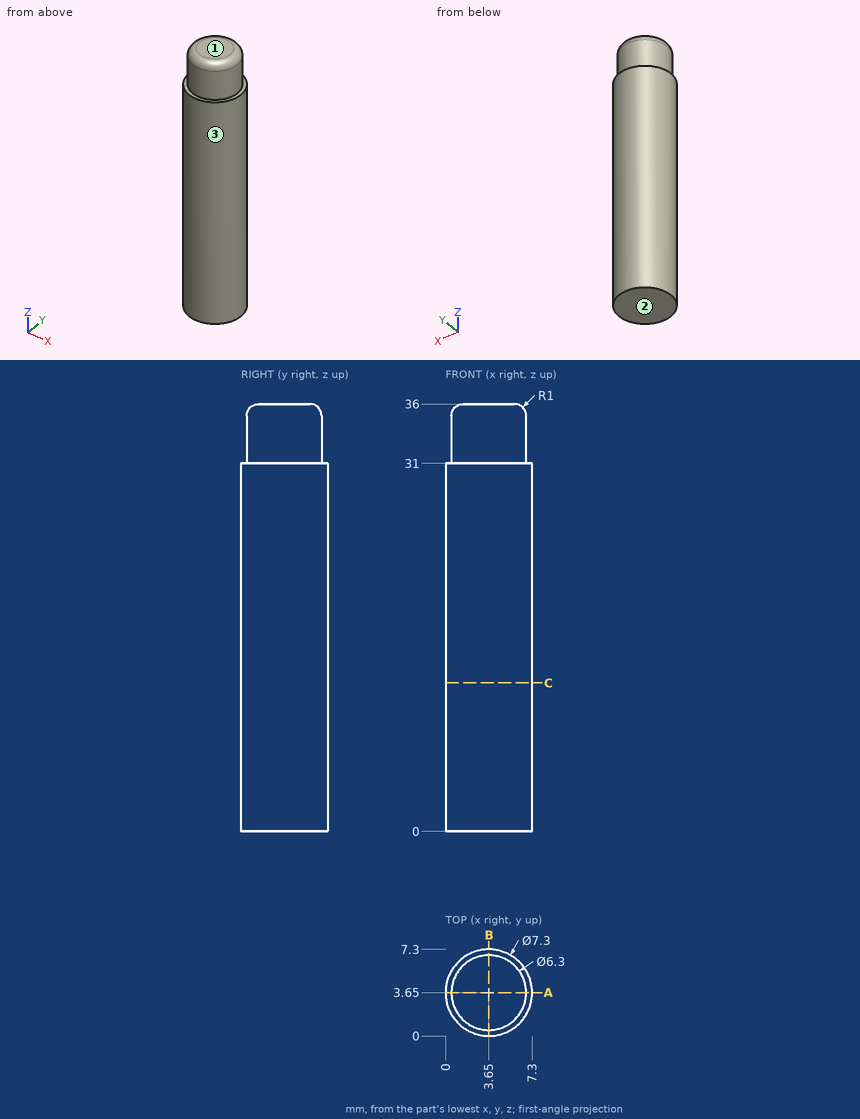
Print and shaded views of the part. All mm, measured from the part's lowest x, y and z. Give positions to 0.01 mm unless a question says otherwise; leave off trailing zeros. Loops run counter-clockwise (first coordinate to the right, second up) from the corner with the lowest first, then second, coordinate; pieces in that order, holes last. Notation, with made-up numbers: (3.25, 14) -> (10.25, 14) arc R6 ccw to (10.25, 20) -> close; hole circle Ø5 at (-30.75, 4.5). An arc over 180 degrees is marked (long way). One line per question, with ' | ' between items. Start each with the question number.
1) Two-plate mould, pull along Z, no slides. Class the marked faces 1, 2 and 3: released by +Z, released by -Z, zero draft, split by the parting line, or undercut.
2) Probe L1, parallel to Y at x = 3.75, z = 27; L2, parallel to Z at x = 1.25, y = 6; L3, parallel to Y at x = 1.5, z = 3. List the from-to ranges inside material, lowest first.
3) Cut at C-C (z = 12.5). Give the cut face in (x, y), plus the area to 3 significant figures.
4) Cut at A-A (y = 3.65). Give the cut face in (x, z), plus the area to 3 significant figures.
Return value:
1) face 1: released by +Z | face 2: released by -Z | face 3: zero draft
2) L1: 0 to 7.3 | L2: 0 to 31 | L3: 0.7 to 6.6
3) outline: circle Ø7.3 at (3.65, 3.65) | area: 41.9 mm^2
4) outline: (0, 0) -> (7.3, 0) -> (7.3, 31) -> (6.8, 31) -> (6.8, 35) arc R1 ccw to (5.8, 36) -> (1.5, 36) arc R1 ccw to (0.5, 35) -> (0.5, 31) -> (0, 31) -> close | area: 257 mm^2
